from build123d import *

# Parameters (mm, degrees)
BOSS_EXTRUDE1_DEPTH = 30
SKETCH2_R           = 1.5
CUT_EXTRUDE1_DEPTH  = 6
SKETCH3_R           = 1.5
BOSS_EXTRUDE2_DEPTH = 6


with BuildPart() as part:
    # Sketch1 → Boss-Extrude1 (new body)
    with BuildSketch(Plane.XY):
        Polygon((0, 2.65), (-2.29496732, 1.325), (-2.29496732, -1.325), (0, -2.65), (2.29496732, -1.325), (2.29496732, 1.325), align=None)
    extrude(amount=BOSS_EXTRUDE1_DEPTH)

    # Sketch2 → Cut-Extrude1 (cut)
    with BuildSketch(Plane(origin=(0, 0, 0), x_dir=(-1, 0, 0), z_dir=(0, 0, -1))):
        Circle(SKETCH2_R)
    extrude(amount=-CUT_EXTRUDE1_DEPTH, mode=Mode.SUBTRACT)

    # Sketch3 → Boss-Extrude2 (add)
    with BuildSketch(Plane.XY.offset(30)):
        with Locations(Location((0, 0, 0), (0, 0, 180))):
            Circle(SKETCH3_R)
    extrude(amount=BOSS_EXTRUDE2_DEPTH)


solid = part.part
Input: part model. Units: mm. Frame: model coordinates. A direction names the side the tool comes from. Give positions to 0.01 mm unless a question says otherwise; leave off trailing zeros. Loops run counter-clockwise (first coordinate to the right, second up) from the corner with the lowest first, then second, coordinate; pieces in that order, holes last. Notation, with made-up numbers: M -29,18 L 28,18 A22 cw 28,30 Z; hole C 78,15 d2. An arc over 180 degrees is marked long. Use one line per item in the form item = value.
1. Section query C-C, the plane x = 0.65. Return the cut outline in (y, z).
Numbers:
outline = M -2.27,0 L -1.35,0 L -1.35,6 L 1.35,6 L 1.35,0 L 2.27,0 L 2.27,30 L 1.35,30 L 1.35,36 L -1.35,36 L -1.35,30 L -2.27,30 Z
2. Line query: L1, parallel to Z at x = -1.1, y = 1.9; L2, parallel to Z at x = -1, y = 1.05; L3, parallel to Y at x = 0.55, z = 3.5. Output: solid intervals per line, ascending.
Numbers:
L1 = 0 to 30
L2 = 6 to 36
L3 = -2.33 to -1.4, 1.4 to 2.33
3. First-contact query: pin 1 (1 mm diameter, centred on y = -1, z = 32, fed in from +X); pin 2 (1.5 mm diameter, centred on x = 0.5, y = 0.5, fed in from -Z). Flat tips, straight axial feed; report the tip coordinate or a pass-through.
Numbers:
pin_1 = 1.41
pin_2 = 6
4. Section query B-B, the plane z = 11. Return the cut outline in (x, y) (3 decimals).
Numbers:
outline = M -2.295,-1.325 L 0,-2.65 L 2.295,-1.325 L 2.295,1.325 L 0,2.65 L -2.295,1.325 Z
5. Section query D-D, the plane y = 1.95. Return the cut outline in (x, z), and give its area (3 significant figures).
Numbers:
outline = M -1.21,0 L 1.21,0 L 1.21,30 L -1.21,30 Z
area = 72.7 mm²
6. Pull-direction query (Y, two-part tool) for faces 4 (the face through (-1.16, -1.98, 14.79)), 5 (the face through (0, 0, 6)), 6 (the face through (-2, 0, 0)); classes: released by +Y, released by -Y, zero draft, split by the parting line, or undercut.
Numbers:
face_4 = released by -Y
face_5 = undercut
face_6 = zero draft
7. Section query A-A, the plane y = 0. Return the cut outline in (x, z), and give its area (3 significant figures).
Numbers:
outline = M -2.29,0 L -1.5,0 L -1.5,6 L 1.5,6 L 1.5,0 L 2.29,0 L 2.29,30 L 1.5,30 L 1.5,36 L -1.5,36 L -1.5,30 L -2.29,30 Z
area = 138 mm²
8. Reachability of faces 1 (the face through (1.5, 0.07, 2.96)), 2 (the face through (2.295, 0, 15)), 3 (the face through (-1.43, -0.45, 32.96)) from +Z, -Z, +X, -X, +Y, -Y: full face, straight path, thin tool, end or side. Return the list, or none.
Numbers:
face_1 = -Z
face_2 = +Z, -Z, +X, +Y, -Y
face_3 = +Z
